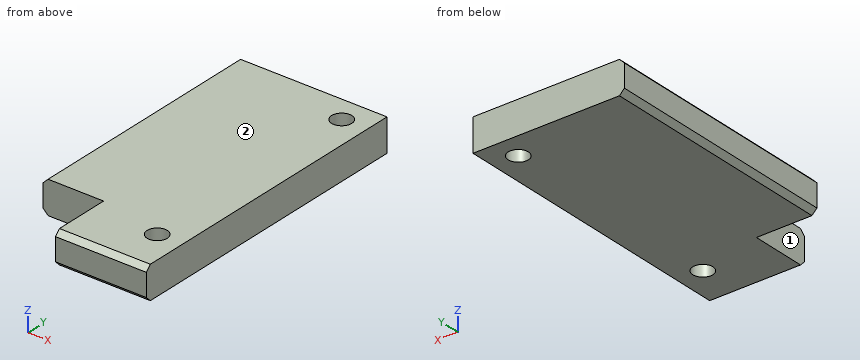
from build123d import *

# Parameters (mm, degrees)
F0_R     = 2
F1_DEPTH = 6.5
F2_SIZE  = 1


# Not quite as in the source:
# - a feature names something its author has since deleted; it is built from what else it names


with BuildPart() as f1:
    # F0 (on Top) → F1 (new body)
    with BuildSketch(Plane.XY):
        Polygon((12, 12), (12, 0), (30, 0), (30, 60), (0, 60), (0, 12), align=None)
        with Locations((25, 9)):
            Circle(F0_R, mode=Mode.SUBTRACT)
        with Locations((25, 55)):
            Circle(F0_R, mode=Mode.SUBTRACT)
    extrude(amount=F1_DEPTH)

    # F2
    f2_edges = [f1.edges().sort_by_distance(p)[0] for p in [
        (21, 0, 0),
        (21, 0, 6.5),
        (0, 36, 0),
        (0, 36, 6.5),
    ]]
    chamfer(f2_edges, length=F2_SIZE)


solid = f1.part
Work out the finished part from the listing and answer in its coordinate system (mm). Face numbers are marked on the shaded views. A direction names the side the tool comes from. Coordinates: 2 decimals unless noted, no trailing zeros. Write each loop counter-clockwise with the first axis right and the second up, starting at its lowest first coordinate (ties: lowest second). Pieces come first, ordered by that corner, then holes. Notation, with made-up numbers: (9, 85.25) - (52, 85.25) arc R26 cw to (52, 124.25) - close; hole circle Ø2 at (28.25, -4). An arc over 180 degrees is marked (long way). One line per question, with ' | ' between items.
1) Consider probe 1 along Y at (x, z) = (25, 1.5); probe 2 along Y at (x, z) = (25.75, 2.5); probe 3 along X at (y, z) = (54, 4.5). Determine where each line is inside the solid, lowest interval first. Write a range as [from, to].
Checks:
probe 1: [0, 7], [11, 53], [57, 60] | probe 2: [0, 7.15], [10.85, 53.15], [56.85, 60] | probe 3: [0, 23.27], [26.73, 30]
2) Find section A-A, the plane x = 25. Determine the outline of the cut face in (y, z).
Checks:
outline: (0, 1) - (1, 0) - (7, 0) - (7, 6.5) - (1, 6.5) - (0, 5.5) - close; (11, 0) - (53, 0) - (53, 6.5) - (11, 6.5) - close; (57, 0) - (60, 0) - (60, 6.5) - (57, 6.5) - close
3) Find section D-D, the plane y = 9. Determine the outline of the cut face in (x, z), and give its area (3 significant figures).
Checks:
outline: (12, 0) - (23, 0) - (23, 6.5) - (12, 6.5) - close; (27, 0) - (30, 0) - (30, 6.5) - (27, 6.5) - close | area: 91.0 mm2
4) Find section C-C, the plane z = 4.75. Determine the outline of the cut face in (x, y).
Checks:
outline: (0, 12) - (12, 12) - (12, 0) - (30, 0) - (30, 60) - (0, 60) - close; hole circle Ø4 at (25, 9); hole circle Ø4 at (25, 55)
5) A flat-ended cylindrical pin translates along its axis: P1, Ø1, axis at x = 9.5, z = 2.5, coming from the -Y side. Find the tip coordinate at first contact, or state that the pin passes through.
Checks:
P1: y = 12
6) For the marked faces 1 and 2, determine the directions among +Z, -Z, +X, -X, +Y, -Y from which every point of the face is accessible in a straight line to the end or side of a thin tool.
Checks:
face 1: +Z, -Z, -X, -Y | face 2: +Z, +X, -X, +Y, -Y
7) Find section B-B, the plane y = 55. Determine the outline of the cut face in (x, z), and give its area (3 significant figures).
Checks:
outline: (0, 1) - (1, 0) - (23, 0) - (23, 6.5) - (1, 6.5) - (0, 5.5) - close; (27, 0) - (30, 0) - (30, 6.5) - (27, 6.5) - close | area: 168 mm2
